from build123d import *

# Parameters (mm, degrees)
SKETCH_1_W      = 1800
SKETCH_1_H      = 2000
EXTRUDE_1_DEPTH = 400
EXTRUDE_2_DEPTH = 60


with BuildPart() as part:
    # 草图1 → 凸台-拉伸1 (new body)
    with BuildSketch(Plane(origin=(0, 0, 0), x_dir=(1, 0, 0), z_dir=(0, 1, 0))):
        with Locations((-900, -1000)):
            Rectangle(SKETCH_1_W, SKETCH_1_H)
    extrude(amount=-EXTRUDE_1_DEPTH)

    # 草图2 → 凸台-拉伸2 (add)
    with BuildSketch(Plane(origin=(0, 0, 0), x_dir=(-1, 0, 0), z_dir=(0, 0, -1))):
        with BuildLine():
            Line((1800, -400), (1800, 500))
            ThreePointArc((1800, 500), (1770.710678119, 570.710678119), (1700, 600))
            Line((1700, 600), (100, 600))
            ThreePointArc((100, 600), (29.289321881, 570.710678119), (0, 500))
            Line((0, 500), (0, -400))
            Line((0, -400), (1800, -400))
        make_face()
    extrude(amount=EXTRUDE_2_DEPTH)


solid = part.part
For this review, take the finished solid that the model builds, in its own axes (mm). A direction names the side the tool comes from. Round coordinates to 2 decimals unless told otherwise and drop trailing zeros. Loops run counter-clockwise (first coordinate to the right, second up) from the corner with the lowest first, then second, coordinate; pieces in that order, holes last. Notation, with made-up numbers: (-29.5, -36.5) - (14.5, -36.5) arc R15 ccw to (14.5, -30.5) - close; hole circle Ø3 at (14, -31). An arc over 180 degrees is marked (long way). Put each result on its own line as item: value. Start each with the question number.
1. Insertion check: P1, Ø3, axis at x = -1023, z = 1108.5, coming from the +Y side; P2, Ø1.5, axis at x = -1130.5, y = 315, coming from the +Z side. Each pin has a flat end and moves straight along its axis. Give the tip position at first contact, or say it passes through.
2. For faces 1 (the flat face through (-887, -400, 984)), 2 (the flat face through (-887, 304, 0)), list the 3-axis set-ups (+Z, -Z, +X, -X, +Y, -Y) from which the entire face can be reached by the end or side of a thin tool; tool diameter is ignored.
3. Consider section C-C on z = 1308.5. State the section outline as (x, y) points, plus the area to 3 significant figures.
4. For probe 1 along Z at (x, y) = (-428, 273.5); probe 2 along Y at (x, z) = (-360.5, 466.5), list the stretches that pass through material, from the lowest coordinate up. Write a range as [from, to].
5. Consider section B-B on x = -374. State the section outline as (y, z) points.
6. Consider section A-A on y = 439. State the section outline as (x, z) points, plus the area to 3 significant figures.
Result sheet:
1. P1: y = 0
1. P2: z = 0
2. face 1: +Z, -Z, +X, -X, -Y
2. face 2: +Z, +X, -X, +Y
3. outline: (-1800, -400) - (0, -400) - (0, 0) - (-1800, 0) - close
3. area: 720,000 mm^2
4. probe 1: [-60, 0]
4. probe 2: [-400, 0]
5. outline: (-400, -60) - (600, -60) - (600, 0) - (0, 0) - (0, 2000) - (-400, 2000) - close
6. outline: (-1800, -60) - (0, -60) - (0, 0) - (-1800, 0) - close
6. area: 108,000 mm^2
